Geometry: final body of the model. Coordinates: model frame, mm. Give positions to 0.01 mm unless a question says otherwise; leave off trailing zeros. Loops run counter-clockwise (first coordinate to the right, second up) from the corner with the lowest first, then second, coordinate; pieces in that order, holes last. Notation, with made-up numbers: (56.5, 2.25) - (76.5, 2.25) arc R33 ccw to (76.5, 39.25) - close; hole circle Ø4 at (-15, -20.5). An arc over 180 degrees is marked (long way). Answer in a Markdown table with one row per item.
from build123d import *

# Parameters (mm, degrees)
F0_W     = 88.9
F0_H     = 1066.8
F1_DEPTH = 19.05
F2_SIZE  = 88.89999
F3_SIZE  = 88.89999


# Not quite as in the source:
# - a fillet or chamfer is up to 0.001 mm smaller than in the source, because OpenCascade refuses the exact size


with BuildPart() as f1:
    # F0 (on Top) → F1 (new body)
    with BuildSketch(Plane.XY):
        with Locations((-52.413374114, 471.9619610548)):
            Rectangle(F0_W, F0_H)
    extrude(amount=F1_DEPTH)

    # F2 (size 88.9 in the source; OpenCascade refuses exactly that, so slightly less here)
    f2_edges = [f1.edges().sort_by_distance(p)[0] for p in [
        (-7.963374, -61.438039, 9.525),
    ]]
    chamfer(f2_edges, length=F2_SIZE)

    # F3 (size 88.9 in the source; OpenCascade refuses exactly that, so slightly less here)
    f3_edges = [f1.edges().sort_by_distance(p)[0] for p in [
        (-7.963374, 1005.361961, 9.525),
    ]]
    chamfer(f3_edges, length=F3_SIZE)


solid = f1.part
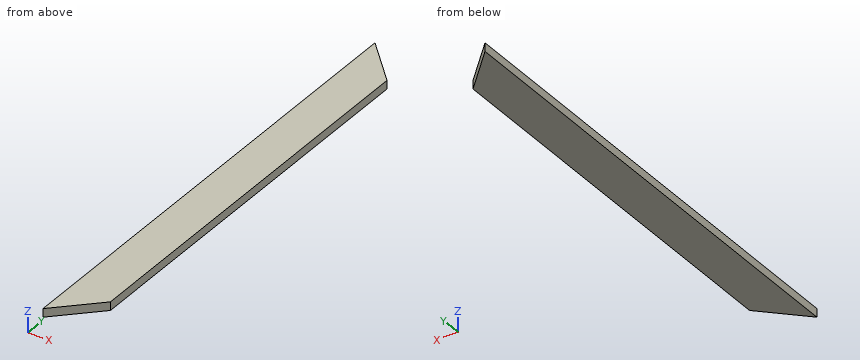
Q1. First-contact query: pin 1 (1 mm diameter, centred on x = -62, y = 775.5, fed in from -Z). Flat tip, straight axial feed; report the tip coordinate or a pass-through.
Check values:
| item | result |
|---|---|
| pin 1 | z = 0 |
Q2. Cut plane C-C (x = -30.5). Output: boundary loops of the cut face in (y, z), and give its area (3 significant figures).
Check values:
| item | result |
|---|---|
| outline | (4.93, 0) - (939, 0) - (939, 19.05) - (4.93, 19.05) - close |
| area | 17,800 mm² |
Q3. Material intervals for line 1 along Y through (x, z) = (-22, 12.75); line 2 along Y through (x, z) = (-36, 8.25); line 3 along X through (y, z) = (-11, 15), sorted ascending.
Check values:
| item | result |
|---|---|
| line 1 | 13.43 to 930.5 |
| line 2 | -0.57 to 944.5 |
| line 3 | -96.86 to -46.43 |
Q4. Cut plane B-B (x = -87.5). Output: boundary loops of the cut face in (y, z).
Check values:
| item | result |
|---|---|
| outline | (-52.07, 0) - (996, 0) - (996, 19.05) - (-52.07, 19.05) - close |
